Can you work these out from the model? Positions are in its coordinate system, mm. A direction names the side the tool comes from. Give positions to 0.01 mm unless a question says otherwise; leave off trailing zeros. Loops run counter-clockwise (first coordinate to the right, second up) from the corner with the lowest first, then second, coordinate; pieces in that order, holes last. Notation, with made-up numbers: M 54,-27.5 L 90,-27.5 A7 ccw 90,-17.5 Z; hole C 13.5,-30 d5. An arc over 180 degrees is marked long. Use CSV: the item, a comma, the result in double quotes.
Autodesk Inventor part; units mm, degrees
ref_plane "YZ Plane" through (0, 0, 0) normal (1, 0, 0) x (0, 1, 0)
ref_plane "XZ Plane" through (0, 0, 0) normal (0, 1, 0) x (-1, 0, 0)
ref_plane "XY Plane" through (0, 0, 0) normal (0, 0, 1) x (1, 0, 0)
sketch "Sketch1" plane through (0, 0, 0) normal (0, 0, 1) x (1, 0, 0)
  line L0 (0, 0) -> (215.9, 0)
  line L1 (215.9, 0) -> (215.9, 139.7)
  line L2 (215.9, 139.7) -> (0, 139.7)
  line L3 (0, 139.7) -> (0, 0)
  dimension "d0" = 215.9
  dimension "d1" = 139.7
extrude "Plate1" add sketch "Sketch1" along normal blind 2.286
sketch "Sketch2" plane through (0, 0, 2.286) normal (0, 0, 1) x (1, 0, 0)
  line L0 (0, 0) -> (0, 139.7)
  line L1 (215.9, 0) -> (0, 0)
  line L2 (215.9, 139.7) -> (215.9, 0)
  line L3 (0, 139.7) -> (215.9, 139.7)
sketch "Sketch3" plane through (0, 0, 2.286) normal (0, 0, 1) x (1, 0, 0)
  line L0 (0, 0) -> (0, 139.7)
  line L1 (215.9, 0) -> (0, 0)
  line L2 (215.9, 139.7) -> (215.9, 0)
  line L3 (0, 139.7) -> (215.9, 139.7)
  line L4 (38.1, 108.0084) -> (38.1, 31.8084)
  line L5 (25.4, 31.8084) -> (25.4, 108.0084)
  arc A0 (38.1, 108.0084) -> (25.4, 108.0084) centre (31.75, 108.0084) ccw
  arc A1 (25.4, 31.8084) -> (38.1, 31.8084) centre (31.75, 31.8084) ccw
  line L6 (127.1585, 108.0084) -> (127.1585, 31.8084)
  line L7 (114.4585, 31.8084) -> (114.4585, 108.0084)
  arc A2 (127.1585, 108.0084) -> (114.4585, 108.0084) centre (120.8085, 108.0084) ccw
  arc A3 (114.4585, 31.8084) -> (127.1585, 31.8084) centre (120.8085, 31.8084) ccw
  line L8 (55.9503, 111.8766) -> (95.9974, 111.8766)
  line L9 (102.0898, 103.1902) -> (73.5837, 24.4878)
  line L10 (55.9503, 99.1766) -> (87.1287, 99.1766)
  line L11 (87.1287, 99.1766) -> (61.6428, 28.8128)
  line L12 (73.5837, 24.4878) -> (73.5837, 24.4878)
  arc A4 (55.9503, 111.8766) -> (55.9503, 99.1766) centre (55.9503, 105.5266) ccw
  arc A5 (61.6428, 28.8128) -> (73.5837, 24.4878) centre (67.6132, 26.6503) ccw
  arc A6 (102.0898, 103.1902) -> (95.9974, 111.8766) centre (95.9974, 105.3969) ccw
  ellipse E0 centre (164.6613, 85.8797) end of major axis (164.6613, 113.2513) minor radius 25.8041 (187.1505, 72.4584) -> (166.8072, 58.6028) ccw
  line L13 (187.1505, 72.4584) -> (162.6138, 25.1653)
  arc A7 (150.6572, 27.4744) -> (162.6138, 25.1653) centre (156.9773, 28.0896) ccw
  line L14 (150.6572, 27.4744) -> (166.8072, 58.6028)
  dimension "d15" = 12.7
  dimension "d16" = 76.2
  dimension "d17" = 12.7
  dimension "d18" = 76.2
  dimension "d19" = 12.7
  dimension "d33" = 6.35
extrude "Cut2" cut sketch "Sketch3" against normal blind 2.286 contours L4 A1 L5 A0 | L6 A3 L7 A2 | L8 A6 L9 A5 L11 L10 A4 | L13 A7 L14 E0
sketch "Sketch4" plane through (0, 0, 2.286) normal (0, 0, 1) x (1, 0, 0)
  line L0 (87.1287, 99.1766) -> (55.9503, 99.1766)
  arc A0 (55.9503, 111.8766) -> (55.9503, 99.1766) centre (55.9503, 105.5266) ccw
  line L1 (55.9503, 111.8766) -> (95.9974, 111.8766)
  arc A1 (102.0898, 103.1902) -> (95.9974, 111.8766) centre (95.9974, 105.3969) ccw
  line L2 (102.0898, 103.1902) -> (73.5837, 24.4878)
  arc A2 (61.6428, 28.8128) -> (73.5837, 24.4878) centre (67.6132, 26.6503) ccw
  line L3 (61.6428, 28.8128) -> (87.1287, 99.1766)
  arc A3 (25.4, 31.8084) -> (38.1, 31.8084) centre (31.75, 31.8084) ccw
  line L4 (25.4, 31.8084) -> (25.4, 108.0084)
  arc A4 (38.1, 108.0084) -> (25.4, 108.0084) centre (31.75, 108.0084) ccw
  line L5 (38.1, 108.0084) -> (38.1, 31.8084)
  arc A5 (114.4585, 31.8084) -> (127.1585, 31.8084) centre (120.8085, 31.8084) ccw
  line L6 (114.4585, 31.8084) -> (114.4585, 108.0084)
  arc A6 (127.1585, 108.0084) -> (114.4585, 108.0084) centre (120.8085, 108.0084) ccw
  line L7 (127.1585, 108.0084) -> (127.1585, 31.8084)
  line L8 (150.6572, 27.4744) -> (166.8072, 58.6028)
  ellipse E0 centre (164.6613, 85.8797) end of major axis (164.6613, 113.2513) minor radius 25.8041 (187.1505, 72.4584) -> (166.8072, 58.6028) ccw
  line L9 (187.1505, 72.4584) -> (162.6138, 25.1653)
  arc A7 (150.6572, 27.4744) -> (162.6138, 25.1653) centre (156.9773, 28.0896) ccw
  line L10 (0, 0) -> (0, 139.7)
  line L11 (215.9, 0) -> (0, 0)
  line L12 (215.9, 139.7) -> (215.9, 0)
  line L13 (0, 139.7) -> (215.9, 139.7)
equation "\"d36\" = Thickness"
equation "\"BendRadius\" = Thickness"
equation "\"BendReliefWidth\" = Thickness"
equation "\"BendReliefDepth\" = 0.5 * Thickness"
equation "\"CornerReliefSize\" = 4 * Thickness"
equation "\"MinimumRemnant\" = 2 * Thickness"
equation "\"TransitionRadius\" = BendRadius"
equation "\"JacobiRadiusSize\" = BendRadius"
equation "\"GapSize\" = Thickness"
equation "\"d2\" = BendRadius"
properties part number "Number Plate"
Q1. I want a section at C-C, the plane z = 1.5. State how many separate pieces and enclosed holes the cut face has, then the cut area to 3 significant figures.
Model answer:
separate pieces,"1"
enclosed holes,"4"
area,"23,600 mm2"
Q2. I want a section at B-B, the plane y = 53.5. Please give me the cut outline in (x, z), then the cut area to 3 significant figures.
Model answer:
outline,"M 0,0 L 25.4,0 L 25.4,2.29 L 0,2.29 Z; M 38.1,0 L 70.58,0 L 70.58,2.29 L 38.1,2.29 Z; M 84.09,0 L 114.46,0 L 114.46,2.29 L 84.09,2.29 Z; M 127.16,0 L 164.16,0 L 164.16,2.29 L 127.16,2.29 Z; M 177.31,0 L 215.9,0 L 215.9,2.29 L 177.31,2.29 Z"
area,"375 mm2"
Q3. Please list where these lines run through material, in increasing order: L1, parallel to X at y = 57, z = 1.9; L2, parallel to X at y = 61, z = 0.55; L3, parallel to Y at x = 163, z = 0.95. Write a range as from..to.
Model answer:
L1,"0..25.4, 38.1..71.85, 85.36..114.46, 127.16..165.98, 179.13..215.9"
L2,"0..25.4, 38.1..73.3, 86.81..114.46, 127.16..153.9, 181.21..215.9"
L3,"0..25.91, 51.26..58.56, 113.19..139.7"
Q4. I want a section at A-A, the plane x = 31.75. Please give me the cut outline in (y, z), then the cut area to 3 significant figures.
Model answer:
outline,"M 0,0 L 25.46,0 L 25.46,2.29 L 0,2.29 Z; M 114.36,0 L 139.7,0 L 139.7,2.29 L 114.36,2.29 Z"
area,"116 mm2"
Q5. For faces 1 (the flat face through (106, 71, 0)), 2 (the cylindrical face through (101.35, 109.05, 1.16)), which set-ups out of +Z, -Z, +X, -X, +Y, -Y let a thin tool reach every point of the face, with its end or its side?
Model answer:
face 1,"-Z, +X, -X, +Y, -Y"
face 2,"+Z, -Z"
Q6. If we mould it in two halves opening along X, with no side actions, what happens to faces 3 (the flat face through (106, 71, 2.286)), 4 (the flat face through (88.036, 64.39, 1.159))? For each: released by +X, released by -X, zero draft, split by the parting line, or undercut.
Model answer:
face 3,"zero draft"
face 4,"undercut"
